Can you work these out from the model? Positions are in its coordinate system, mm. A direction names the side the tool comes from. Round coordinates to 2 decimals unless told otherwise and drop trailing zeros. Order: outer loops, then holes, each group sorted by start corner. A loop starts at its lowest first (then second) coordinate and runs counter-clockwise, first axis right, second up. Notation, with made-up numbers: (11, 66.25) -> (41, 66.25) arc R34 ccw to (41, 101.25) -> close; hole circle Ø10 at (50, 45). An arc over 180 degrees is marked (long way). One line per item, written item: value.
```python
from build123d import *


with BuildPart() as f1:
    # F0 (on Top) → F1 (revolve)
    with BuildSketch(Plane.XY):
        with BuildLine():
            ThreePointArc((2.828427, -156.103516), (0, -154.931943), (-2.828427, -156.103516))
            Line((-2.828427, -156.103516), (-10.828427, -164.103516))
            ThreePointArc((-10.828427, -164.103516), (-11.695518, -165.40121), (-12, -166.931943))
            Line((-12, -166.931943), (-12, -176.931943))
            ThreePointArc((-12, -176.931943), (0, -203.2), (12, -176.931943))
            Line((12, -176.931943), (12, -166.931943))
            ThreePointArc((12, -166.931943), (11.695518, -165.40121), (10.828427, -164.103516))
            Line((10.828427, -164.103516), (2.828427, -156.103516))
        make_face()
    revolve(axis=Axis((-7.103204, 0, 0), (-1, 0, 0)))


solid = f1.part
```
Q1. Please list where these lines run through material, in increasing order: line 1 along X through (y, z) = (-29, -165); line 2 along Z through (x, y) = (-13, 1); line 3 along Z through (x, y) = (-8.5, -117.5).
Answers below:
line 1: -12 to 12
line 2: -196.43 to -178.21, 178.21 to 196.43
line 3: -162.75 to -111.2, 111.2 to 162.75
Q2. Will these pins go through, and if not, where does the flat tip stop? pin 1 Ø4 at (x, y) = (10, -123.5) entering from -Z; pin 2 Ø10 at (x, z) = (0.5, -117) entering from +Y; pin 3 Ø10 at (x, z) = (3, 156.5) entering from -Y.
Answers below:
pin 1: z = -159.27
pin 2: y = 169.54
pin 3: y = -135.12
Q3. On a 3-axis mill with a long thin cutter (end or side, diameter ignored), from which of +Z, -Z, +X, -X, +Y, -Y can I reach the whole of each face in a straight line? I mean faces 1 (the face through (-12, 130, 106)), 2 (the face through (12, -130, 106)). Say none if no direction works.
Answers below:
face 1: -X
face 2: +X
Q4. I want a section at A-A on y = 0. List the corners of the cut face in (x, z) for me (3 decimals).
Answers below:
outline: (-12, -176.932) arc R15.875 ccw (long way) to (12, -176.932) -> (12, -166.932) arc R4 ccw to (10.828, -164.104) -> (2.828, -156.104) arc R4 ccw to (-2.828, -156.104) -> (-10.828, -164.104) arc R4 ccw to (-12, -166.932) -> close; (-12, 166.932) arc R4 ccw to (-10.828, 164.104) -> (-2.828, 156.104) arc R4 ccw to (2.828, 156.104) -> (10.828, 164.104) arc R4 ccw to (12, 166.932) -> (12, 176.932) arc R15.875 ccw (long way) to (-12, 176.932) -> close
